from build123d import *

# Parameters (mm, degrees)
F1_DEPTH = 1.524
F0_W     = 38.1
F0_H     = 101.996876
F0_R     = 2.3114
F2_DEPTH = 2.667


with BuildPart() as f1:
    # F0 (on Right) → F1 (new body)
    with BuildSketch(Plane.YZ):
        Polygon((0, 69.949219), (0, 88.9), (-27.94, 88.9), (-30.48, 93.98), (-33.02, 83.82), (-35.56, 88.9), (-63.5, 88.9), (-63.5, -88.9), (-35.56, -88.9), (-33.02, -93.98), (-30.48, -83.82), (-27.94, -88.9), (0, -88.9), (0, -69.949219), (-50.8, -69.949219), (-50.8, 69.949219), align=None)
        Polygon((0, 50.998438), (0, 69.949219), (-50.8, 69.949219), (-50.8, -69.949219), (0, -69.949219), (0, -50.998438), (-38.1, -50.998438), (-38.1, 50.998438), align=None)
    extrude(amount=F1_DEPTH)

    # F0 (on Right) → F2 (join)
    with BuildSketch(Plane.YZ):
        Polygon((0, 50.998438), (0, 69.949219), (-50.8, 69.949219), (-50.8, -69.949219), (0, -69.949219), (0, -50.998438), (-38.1, -50.998438), (-38.1, 50.998438), align=None)
        with Locations((-19.05, 0)):
            Rectangle(F0_W, F0_H)
        with Locations((-18.851562, -38.1)):
            Circle(F0_R, mode=Mode.SUBTRACT)
        with Locations((-28.376562, -12.7)):
            Circle(F0_R, mode=Mode.SUBTRACT)
        with Locations((-28.376562, 12.7)):
            Circle(F0_R, mode=Mode.SUBTRACT)
        with Locations((-18.851562, 38.1)):
            Circle(F0_R, mode=Mode.SUBTRACT)
    extrude(amount=-F2_DEPTH)


solid = f1.part
The model under review builds one solid part; all positions refer to its coordinate system, in mm. A direction names the side the tool comes from. Coordinates: 2 decimals unless noted, no trailing zeros. Write each loop counter-clockwise with the first axis right and the second up, starting at its lowest first coordinate (ties: lowest second). Pieces come first, ordered by that corner, then holes. Notation, with made-up numbers: M 10,87 L 36,87 A14 cw 36,98 Z; hole C 22,7.5 d2. An arc over 180 degrees is marked long. Put each result on its own line as item: value.
1) Add section C-C on y = -4. Give the boundary of the cut face in (x, z).
Computed:
outline: M -2.67,-69.95 L 0,-69.95 L 0,-88.9 L 1.52,-88.9 L 1.52,-51 L 0,-51 L 0,51 L 1.52,51 L 1.52,88.9 L 0,88.9 L 0,69.95 L -2.67,69.95 Z
2) Clearance check with flat-ended pins moving along their axes: pin 1 Ø1.2 at (x, y) = (0.5, -52.5) entering from +Z; pin 2 Ø0.8 at (x, z) = (0.5, 5.5) entering from +Y; pin 3 Ø0.8 at (x, z) = (-2, -2.5) entering from -Y; pin 4 Ø3.5 at (y, z) = (-18.85, -38.1) entering from -X. State where each tip first meets the part, or that it passes through.
Computed:
pin 1: stops at z = 88.9
pin 2: stops at y = -38.1
pin 3: stops at y = -50.8
pin 4: passes through
3) For faces 4 (the flat face through (0, -53, 1)), 5 (the flat face through (0, -19, 1)), 6 (the cylindrical face through (-1.315, -16.647, 38.794)), list the 3-axis set-ups (+Z, -Z, +X, -X, +Y, -Y) from which the entire face can be reached by the end or side of a thin tool; tool diameter is ignored.
Computed:
face 4: -X, -Y
face 5: +X, +Y
face 6: +X, -X
4) Wall thickness on probe 1 along Z at (x, y) = (1.3, -3.5); probe 2 along X at (y, z) = (-21.5, 14); probe 3 along Y at (x, z) = (0.25, 22): over which ranges is each line inside the solid? List them lowest first. Write a range as [from, to].
Computed:
probe 1: z = [-88.9, -51], [51, 88.9]
probe 2: x = [-2.67, 0]
probe 3: y = [-63.5, -38.1]
5) Draft analysis for pull direction Z (two halves, no side actions). For faces 1 (the cylindrical face through (-1.31, -26.17, -12.01)), 2 (the flat face through (1.524, -39, 1)), 3 (the cylindrical face through (-1.31, -17.61, -36.15)), state which applies: released by +Z, released by -Z, zero draft, split by the parting line, or undercut.
Computed:
face 1: undercut
face 2: zero draft
face 3: undercut
6) Add section A-A on z = 38.1. Give the boundary of the cut face in (x, y), then the cut area to 3 significant figures.
Computed:
outline: M -2.67,-50.8 L 0,-50.8 L 0,-63.5 L 1.52,-63.5 L 1.52,-38.1 L 0,-38.1 L 0,-21.16 L -2.67,-21.16 Z; M -2.67,-16.54 L 0,-16.54 L 0,0 L -2.67,0 Z
area: 162 mm2
7) Add section B-B on x = -1. Give the boundary of the cut face in (y, z), then the cut area to 3 significant figures.
Computed:
outline: M -50.8,-69.95 L 0,-69.95 L 0,69.95 L -50.8,69.95 Z; hole C -28.38,-12.7 d4.62; hole C -28.38,12.7 d4.62; hole C -18.85,-38.1 d4.62; hole C -18.85,38.1 d4.62
area: 7,040 mm2
8) Add section D-D on z = -78.5. Give the boundary of the cut face in (x, y).
Computed:
outline: M 0,-63.5 L 1.52,-63.5 L 1.52,0 L 0,0 Z
